from build123d import *

# Parameters (mm, degrees)
SKETCH1_W           = 38
SKETCH1_H           = 32.3
SKETCH1_W_2         = 24
SKETCH1_H_2         = 13
BOSS_EXTRUDE1_DEPTH = 1.4
SKETCH2_R           = 1.3
BOSS_EXTRUDE2_DEPTH = 4
FILLET1_R           = 1.5


with BuildPart() as part:
    # Sketch1 → Boss-Extrude1 (new body)
    with BuildSketch(Plane(origin=(0, 0, 0), x_dir=(1, 0, 0), z_dir=(0, 1, 0))):
        with Locations((0, -1.65)):
            Rectangle(SKETCH1_W, SKETCH1_H)
        Rectangle(SKETCH1_W_2, SKETCH1_H_2, mode=Mode.SUBTRACT)
    extrude(amount=BOSS_EXTRUDE1_DEPTH)

    # Sketch2 → Boss-Extrude2 (add)
    with BuildSketch(Plane(origin=(0, 1.4, 0), x_dir=(1, 0, 0), z_dir=(0, 1, 0))):
        with Locations(Location((-10.25, 10, 0), (0, 0, 270))):
            Circle(SKETCH2_R)
        with Locations(Location((-10.25, -13.5, 0), (0, 0, 270))):
            Circle(SKETCH2_R)
        with Locations(Location((10.25, -13.5, 0), (0, 0, 90))):
            Circle(SKETCH2_R)
        with Locations(Location((10.25, 10, 0), (0, 0, 90))):
            Circle(SKETCH2_R)
    extrude(amount=BOSS_EXTRUDE2_DEPTH)

    # Fillet1
    fillet1_edges = [part.edges().sort_by_distance(p)[0] for p in [
        (-10.25, 1.4, -11.3),
        (-10.25, 1.4, 12.2),
        (10.25, 1.4, 14.8),
        (10.25, 1.4, -8.7),
    ]]
    fillet(fillet1_edges, radius=FILLET1_R)


solid = part.part
Here's how the part is built. I have some questions about the finished solid (model axes, mm). A direction names the side the tool comes from. Coordinates: 2 decimals unless noted, no trailing zeros. Loops run counter-clockwise (first coordinate to the right, second up) from the corner with the lowest first, then second, coordinate; pieces in that order, holes last. Notation, with made-up numbers: (10, 42.25) -> (36, 42.25) arc R18 ccw to (36, 73.25) -> close; hole circle Ø4 at (-2.5, 48). An arc over 180 degrees is marked (long way). Use one line per item in the form item = value. Start each with the question number.
(1) Please list where these lines run through material, in increasing order: line 1 along X through (y, z) = (0.55, 1); line 2 along Y through (x, z) = (-13, -9.5); line 3 along Z through (x, y) = (-8, 0.7).
(2) Will these pins go through, and if not, where does the flat tip stop? pin 1 (12 mm diameter, centred on x = -4, z = -8.5, fed in from +Y); pin 2 (2 mm diameter, centred on y = 3, z = -8.5, fed in from +X); pin 3 (10 mm diameter, centred on x = 0.5, z = 11, fed in from +Y); pin 4 (1.5 mm diameter, centred on x = -11.5, y = 3.5, fed in from +Z).
(3) If we section it at B-B (x = -2): Please give me the cut outline in (y, z), then the cut area to 3 significant figures.
(4) If we section it at A-A (z = 5): Please give me the cut outline in (x, y), then the cut area to 3 significant figures.
(5) We'd pull the mould along Z, two halves only. Please class faces 1 (the face through (0, 1, -14.5)), 2 (the face through (10, 5.4, 14)), 3 (the face through (0, 1, 6.5)): pulls with the +Z half, pulls with the -Z half, needs draft (parallel to the pull), parting line crosses it, or undercut.
(6) If we section it at D-D (z = 13.5): Please give me the cut outline in (x, y), then the cut area to 3 significant figures.
(7) If we section it at C-C (y = 4.1): Please give me the cut outline in (x, z), then the cut area to 3 significant figures.
(8) On a 3-axis mill with a long thin cutter (end or side, diameter ignored), from which of +Z, -Z, +X, -X, +Y, -Y can I reach the whole of each face in a straight line? I mean faces 4 (the face through (-12, 1, 0)), 5 (the face through (-8.96, 4.13, 13.33)), 6 (the face through (-10, 5.4, 13)). Say none if no direction works.
Verdict:
q1.line_1 = -19 to -12, 12 to 19
q1.line_2 = 0 to 1.4
q1.line_3 = -14.5 to -6.5, 6.5 to 17.8
q2.pin_1 = 5.4
q2.pin_2 = 11.45
q2.pin_3 = 1.4
q2.pin_4 = 14.7
q3.outline = (0, -14.5) -> (1.4, -14.5) -> (1.4, -6.5) -> (0, -6.5) -> close; (0, 6.5) -> (1.4, 6.5) -> (1.4, 17.8) -> (0, 17.8) -> close
q3.area = 27.0 mm²
q4.outline = (-19, 0) -> (-12, 0) -> (-12, 1.4) -> (-19, 1.4) -> close; (12, 0) -> (19, 0) -> (19, 1.4) -> (12, 1.4) -> close
q4.area = 19.6 mm²
q5.face_1 = pulls with the -Z half
q5.face_2 = needs draft
q5.face_3 = undercut
q6.outline = (-19, 0) -> (19, 0) -> (19, 1.4) -> (13.05, 1.4) arc R1.5 cw to (11.55, 2.9) -> (11.55, 5.4) -> (8.95, 5.4) -> (8.95, 2.9) arc R1.5 cw to (7.45, 1.4) -> (-7.45, 1.4) arc R1.5 cw to (-8.95, 2.9) -> (-8.95, 5.4) -> (-11.55, 5.4) -> (-11.55, 2.9) arc R1.5 cw to (-13.05, 1.4) -> (-19, 1.4) -> close
q6.area = 75.9 mm²
q7.outline = circle Ø2.6 at (-10.25, -10); circle Ø2.6 at (-10.25, 13.5); circle Ø2.6 at (10.25, -10); circle Ø2.6 at (10.25, 13.5)
q7.area = 21.2 mm²
q8.face_4 = +Y, -Y
q8.face_5 = +Y
q8.face_6 = +Z, -Z, +X, -X, +Y
